from build123d import *

# Parameters (mm, degrees)
BOSS_EXTRUDE1_DEPTH = 3.175
SKETCH2_R           = 1.7272
CUT_EXTRUDE1_DEPTH  = 195.021684248
FILLET1_R           = 12.7


with BuildPart() as part:
    # Sketch1 → Boss-Extrude1 (new body)
    with BuildSketch(Plane(origin=(0, 0, 0), x_dir=(1, 0, 0), z_dir=(0, 1, 0))):
        Polygon((0, 146.646968374), (-127, -73.323484187), (127, -73.323484187), align=None)
    extrude(amount=BOSS_EXTRUDE1_DEPTH)

    # Sketch2 → Cut-Extrude1 (cut, through all)
    with BuildSketch(Plane(origin=(0, 3.175, 0), x_dir=(1, 0, 0), z_dir=(0, 1, 0))):
        with Locations(Location((71.193145986, -32.861822377, 0), (0, 0, 270))):
            Circle(SKETCH2_R)
        with Locations(Location((75.155545986, -25.998744257, 0), (0, 0, 270))):
            Circle(SKETCH2_R)
        with Locations(Location((-64.055745986, -45.224161811, 0), (0, 0, 270))):
            Circle(SKETCH2_R)
        with Locations(Location((-60.093345986, -52.08723993, 0), (0, 0, 270))):
            Circle(SKETCH2_R)
        with Locations(Location((-7.1374, 78.085984187, 0), (0, 0, 270))):
            Circle(SKETCH2_R)
        with Locations(Location((-15.0622, 78.085984187, 0), (0, 0, 270))):
            Circle(SKETCH2_R)
    extrude(amount=-CUT_EXTRUDE1_DEPTH, mode=Mode.SUBTRACT)

    # Fillet1
    fillet1_edges = [part.edges().sort_by_distance(p)[0] for p in [
        (127, 1.5875, 73.323484187),
        (-127, 1.5875, 73.323484187),
        (0, 1.5875, -146.646968374),
    ]]
    fillet(fillet1_edges, radius=FILLET1_R)


solid = part.part
Verification items for the finished model (mm, model axes). Round coordinates to 2 decimals unless told otherwise and drop trailing zeros. Loops run counter-clockwise (first coordinate to the right, second up) from the corner with the lowest first, then second, coordinate; pieces in that order, holes last. Notation, with made-up numbers: M 69.5,45 L 100.5,45 A18 cw 100.5,79 Z; hole C 4,-7 d1. An arc over 180 degrees is marked long. Write each question's results on one line, items separated by ' | '.
1) Scan lines: L1, parallel to Z at x = -1, y = 0.85; L2, parallel to Z at x = -16.5, y = 2.4; L3, parallel to Z at x = -15.5, y = 0.85. Record each from-to range of solid material in increasing order. Write a range as from..to.
Checks:
L1: z = -133.91..73.32 | L2: z = -118.07..-79.04, -77.13..73.32 | L3: z = -119.8..-79.76, -76.42..73.32
2) Gauge pin test, flat end, axial feed: P1, Ø1, axis at y = 2.5, z = -62.5, coming from the +X side. Record the tip position at first contact, or that the pin passes through.
Checks:
P1: stops at x = 48.87
3) Section check B-B on z = -96.5. Record the boundary of the cut face in (x, y) (3 decimals).
Checks:
outline: M -28.952,0 L 28.952,0 L 28.952,3.175 L -28.952,3.175 Z
4) Section check A-A on y = 1.2. Record the boundary of the cut face in (x, z).
Checks:
outline: M -116,54.27 L -11,-127.6 A12.7 ccw 11,-127.6 L 116,54.27 A12.7 ccw 105,73.32 L -105,73.32 A12.7 ccw Z; hole C -64.06,45.22 d3.45; hole C -60.09,52.09 d3.45; hole C -15.06,-78.09 d3.45; hole C -7.14,-78.09 d3.45; hole C 71.19,32.86 d3.45; hole C 75.16,26 d3.45
5) Section check C-C on x = -102. Record the boundary of the cut face in (y, z) (3 decimals).
Checks:
outline: M 0,30.022 L 3.175,30.022 L 3.175,73.323 L 0,73.323 Z
